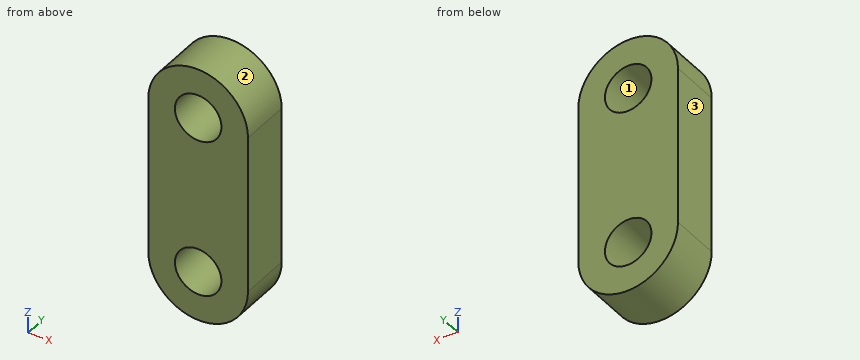
Autodesk Inventor part; units mm, degrees
ref_plane "YZ Plane" through (0, 0, 0) normal (1, 0, 0) x (0, 1, 0)
ref_plane "XZ Plane" through (0, 0, 0) normal (0, 1, 0) x (-1, 0, 0)
ref_plane "XY Plane" through (0, 0, 0) normal (0, 0, 1) x (1, 0, 0)
sketch "Sketch1" plane through (0, 0, 0) normal (0, 1, 0) x (-1, 0, 0)
  line L0 (3, 0) -> (3, 0)
  line L1 (6, -3) -> (6, -12.525)
  line L2 (3, -15.525) -> (3, -15.525)
  line L3 (0, -12.525) -> (0, -3)
  arc A0 (6, -3) -> (3, 0) centre (3, -3) ccw
  arc A1 (3, 0) -> (0, -3) centre (3, -3) ccw
  arc A2 (3, -15.525) -> (6, -12.525) centre (3, -12.525) ccw
  arc A3 (0, -12.525) -> (3, -15.525) centre (3, -12.525) ccw
  circle A4 centre (3, -3) radius 1.4
  circle A5 centre (3, -12.525) radius 1.4
  point P0 (0, 0)
  point P1 (6, -15.525)
  point P2 (6, 0)
  point P3 (0, -15.525)
  dimension "d0" = 6
  dimension "d1" = 15.525
  dimension "d2" = 3
  dimension "d3" = 2.8
  dimension "d4" = 2.8
extrude "Extrusion1" add sketch "Sketch1" along normal blind 3
properties part number "tracks_outer"
Geometry: final body of the model. Coordinates: model frame, mm. Face numbers are marked on the shaded views. Coordinates: 2 decimals unless noted, no trailing zeros. Order: outer loops, then holes, each group sorted by start corner. A loop starts at its lowest first (then second) coordinate and runs counter-clockwise, first axis right, second up.
1) First-contact query: P1, Ø1.5, axis at x = -1, y = 1.5, coming from the +Z side; P2, Ø2.5, axis at x = -3, z = -12.525, coming from the -Y side; P3, Ø1, axis at x = -4, y = 0.5, coming from the -Z side; P4, Ø1, axis at x = -2, y = 1, coming from the +Z side. Flat tips, straight axial feed; report the tip coordinate or a pass-through.
Result sheet:
P1: stops at z = -0.27
P2: passes through
P3: stops at z = -15.48
P4: stops at z = -0.04
2) Section B-B (y = 0.5). Return loops of the section in (x, z) (3 decimals), then the cut area to 3 significant figures.
Result sheet:
outline: (-6, -12.525) arc R3 ccw to (0, -12.525) - (0, -3) arc R3 ccw to (-6, -3) - close; hole circle Ø2.8 at (-3, -12.525); hole circle Ø2.8 at (-3, -3)
area: 73.1 mm2
3) Section A-A (x = -3). Return loops of the section in (y, z) (3 decimals).
Result sheet:
outline: (0, -15.525) - (3, -15.525) - (3, -13.925) - (0, -13.925) - close; (0, -11.125) - (3, -11.125) - (3, -4.4) - (0, -4.4) - close; (0, -1.6) - (3, -1.6) - (3, 0) - (0, 0) - close
4) Section D-D (x = -0.55). Return loops of the section in (y, z).
Result sheet:
outline: (0, -14.26) - (3, -14.26) - (3, -1.27) - (0, -1.27) - close
5) Section C-C (z = -2.25). Return loops of the section in (x, y), then the cut area to 3 significant figures.
Result sheet:
outline: (-5.9, 0) - (-4.18, 0) - (-4.18, 3) - (-5.9, 3) - close; (-1.82, 0) - (-0.1, 0) - (-0.1, 3) - (-1.82, 3) - close
area: 10.3 mm2
6) Draft query along X for the marked faces 1, 2 and 3. Return one class per face: released by +X, released by -X, zero draft, split by the parting line, or undercut.
Result sheet:
face 1: undercut
face 2: split by the parting line
face 3: released by -X
7) Ray query, probe 1 along Z at (x, y) = (-3, 2.2) (3 decimals); probe 2 along Z at (x, y) = (-1.8, 0.9); probe 3 along Z at (x, y) = (-4.55, 0.1). Return the intervals inside material, ascending.
Result sheet:
probe 1: z = -15.525 to -13.925, -11.125 to -4.4, -1.6 to 0
probe 2: z = -15.27 to -13.25, -11.8 to -3.72, -2.28 to -0.25
probe 3: z = -15.09 to -0.43
